from build123d import *

# Parameters (mm, degrees)
SKETCH2_R                      = 4
BOSS_EXTRUDE1_DEPTH            = 110
F_8_0_199_DIAMETER_HOLE3_D     = 5.0546
F_8_0_199_DIAMETER_HOLE3_DEPTH = 10
F_8_0_199_DIAMETER_HOLE3_TIP   = 1.518555042
F_8_0_199_DIAMETER_HOLE4_D     = 5.0546
F_8_0_199_DIAMETER_HOLE4_DEPTH = 10
F_8_0_199_DIAMETER_HOLE4_TIP   = 1.518555042


with BuildPart() as part:
    # Sketch2 → Boss-Extrude1 (new body)
    with BuildSketch(Plane(origin=(0, 0, 0), x_dir=(1, 0, 0), z_dir=(0, 1, 0))):
        Circle(SKETCH2_R)
    extrude(amount=-BOSS_EXTRUDE1_DEPTH)

    # #8 (0.199) Diameter Hole3
    with Locations(Plane(origin=(0, 0, 0), x_dir=(1, 0, 0), z_dir=(0, 1, 0))):
        with Locations((0, 0)):
            Hole(F_8_0_199_DIAMETER_HOLE3_D / 2, depth=F_8_0_199_DIAMETER_HOLE3_DEPTH)
            with Locations((0, 0, -(F_8_0_199_DIAMETER_HOLE3_DEPTH + F_8_0_199_DIAMETER_HOLE3_TIP / 2))):  # 118° drill point
                Cone(0, F_8_0_199_DIAMETER_HOLE3_D / 2, F_8_0_199_DIAMETER_HOLE3_TIP, mode=Mode.SUBTRACT)

    # #8 (0.199) Diameter Hole4
    with Locations(Plane(origin=(0, -110, 0), x_dir=(-1, 0, 0), z_dir=(0, -1, 0))):
        with Locations((0, 0)):
            Hole(F_8_0_199_DIAMETER_HOLE4_D / 2, depth=F_8_0_199_DIAMETER_HOLE4_DEPTH)
            with Locations((0, 0, -(F_8_0_199_DIAMETER_HOLE4_DEPTH + F_8_0_199_DIAMETER_HOLE4_TIP / 2))):  # 118° drill point
                Cone(0, F_8_0_199_DIAMETER_HOLE4_D / 2, F_8_0_199_DIAMETER_HOLE4_TIP, mode=Mode.SUBTRACT)


solid = part.part
Source: CAD feature listing. Evaluate the final solid. Frame: model axes, mm. Coordinates: 2 decimals unless noted, no trailing zeros. Loops run counter-clockwise (first coordinate to the right, second up) from the corner with the lowest first, then second, coordinate; pieces in that order, holes last. Notation, with made-up numbers: (17, 74.5) -> (30, 74.5) arc R17 ccw to (30, 81.5) -> close; hole circle Ø1 at (38.5, 66). An arc over 180 degrees is marked (long way). Answer in a Markdown table with one row per item. Add a question column.
Q1. Pull-direction query (Z, two-part tool) for faces 1 (the face through (-0.867, -54.23, 3.905)), 2 (the face through (-0.548, -104.93, 2.467)), 3 (the face through (0.548, -5.07, 2.467)), 4 (the face through (3, -110, 0)); classes: pulls with the +Z half, pulls with the -Z half, needs draft (parallel to the pull), parting line crosses it, or undercut.
Q2. Ray query, line 1 along Z through (x, y) = (0, -5.5); line 2 along X through (y, z) = (-74, -2.5). Return the intervals inside material, ascending.
Q3. Contact query for flat-ended pins moving along their axis: pin 1 Ø1.5 at (x, y) = (-2.5, -58) entering from +Z; pin 2 Ø1 at (x, z) = (0, -1.5) entering from -Y. Output: stop coordinate, or through.
Q4. Section A-A on y = -17.5. Return the cut outline in (x, z), and give its area (3 significant figures).
Computed values:
| question | item | result |
|---|---|---|
| 1 | face 1 | parting line crosses it |
| 1 | face 2 | undercut |
| 1 | face 3 | undercut |
| 1 | face 4 | needs draft |
| 2 | line 1 | z = -4 to -2.53, 2.53 to 4 |
| 2 | line 2 | x = -3.12 to 3.12 |
| 3 | pin 1 | stops at z = 3.6 |
| 3 | pin 2 | stops at y = -99.68 |
| 4 | outline | circle Ø8 at (0, 0) |
| 4 | area | 50.3 mm^2 |
